from build123d import *

# Parameters (mm, degrees)
SKETCH_1_R                = 30
EXTRUDE_1_DEPTH           = 8
HOLE_WIZARD_2_AT_2_COUNT  = 2
HOLE_WIZARD_2_AT_2_PITCH  = 24
MM_1_D                    = 3
HOLE_WIZARD_3_D           = 4.5
HOLE_WIZARD_3_CBORE_D     = 8
HOLE_WIZARD_3_CBORE_DEPTH = 4.6


with BuildPart() as part:
    # 草图1 → 凸台-拉伸1 (new body)
    with BuildSketch(Plane.XY):
        Circle(SKETCH_1_R)
    extrude(amount=EXTRUDE_1_DEPTH)

    # 草图10 → 打孔尺寸(%根据)内六角圆柱头螺钉的类型2 (revolve, cut)
    with BuildSketch(Plane.YZ.offset(12)):
        Polygon((0, 0), (0, 8), (2.25, 8), (2.25, 4.6), (4, 4.6), (4, 0.025), (4.025, 0), align=None)
    hole_wizard_2 = revolve(axis=Axis((12, 0, -6.35), (0, 0, 1)), mode=Mode.SUBTRACT)

    # 打孔尺寸(%根据)内六角圆柱头螺钉的类型2 at 2: 打孔尺寸(%根据)内六角圆柱头螺钉的类型2 ×2
    with Locations(*[(-i * HOLE_WIZARD_2_AT_2_PITCH, 0, 0) for i in range(1, HOLE_WIZARD_2_AT_2_COUNT)]):
        add(hole_wizard_2, mode=Mode.SUBTRACT)

    # 大小mm 暗销孔1 (through all)
    with Locations(Plane(origin=(0, 0, 0), x_dir=(-1, 0, 0), z_dir=(0, 0, -1))):
        with Locations((0, -17), (0, 17)):
            Hole(MM_1_D / 2)

    # 打孔尺寸(%根据)内六角圆柱头螺钉的类型3 (through all)
    with Locations(Plane.XY.offset(8)):
        with Locations((-20.673237657, 7.524443153), (-20.673237657, -7.524443153), (20.673237657, 7.524443153), (20.673237657, -7.524443153)):
            CounterBoreHole(HOLE_WIZARD_3_D / 2, HOLE_WIZARD_3_CBORE_D / 2, HOLE_WIZARD_3_CBORE_DEPTH)


solid = part.part
Geometry: final body of the model. Coordinates: model frame, mm. A direction names the side the tool comes from. Coordinates: 2 decimals unless noted, no trailing zeros. Write each loop counter-clockwise with the first axis right and the second up, starting at its lowest first coordinate (ties: lowest second). Pieces come first, ordered by that corner, then holes. Notation, with made-up numbers: (-25, 73) - (2, 73) arc R15 cw to (2, 86) - close; hole circle Ø4 at (-25, 7). An arc over 180 degrees is marked (long way). Return JSON: item names as keys, results as strings.
Item 1: Line query: L1, parallel to X at y = 8, z = 3; L2, parallel to X at y = 9.5, z = 1.5; L3, parallel to Y at x = 17, z = 4.75. Output: solid intervals per line, ascending.
Completed:
{"L1": "x = -28.91 to -22.87, -18.47 to 18.47, 22.87 to 28.91", "L2": "x = -28.46 to -21.75, -19.6 to 19.6, 21.75 to 28.46", "L3": "y = -24.72 to -9.11, -5.94 to 5.94, 9.11 to 24.72"}
Item 2: Section query A-A (y = 0). Output: boundary loops of the cut face in (x, z) (3 decimals), and give its area (3 significant figures).
Completed:
{"outline": "(-30, 0) - (-16.025, 0) - (-16, 0.025) - (-16, 4.6) - (-14.25, 4.6) - (-14.25, 8) - (-30, 8) - close; (-9.75, 4.6) - (-8, 4.6) - (-8, 0.025) - (-7.975, 0) - (7.975, 0) - (8, 0.025) - (8, 4.6) - (9.75, 4.6) - (9.75, 8) - (-9.75, 8) - close; (14.25, 4.6) - (16, 4.6) - (16, 0.025) - (16.025, 0) - (30, 0) - (30, 8) - (14.25, 8) - close", "area": "376 mm2"}
Item 3: Reachability of faces 1 (the face through (-15.966, -0.521, 2.28)), 2 (the face through (-16.86, -6.32, 5.73)), 3 (the face through (-0.195, -15.513, 4.056)) from +Z, -Z, +X, -X, +Y, -Y: full face, straight path, thin tool, end or side. Return the list, or none.
Completed:
{"face 1": "-Z", "face 2": "+Z", "face 3": "+Z, -Z"}
Item 4: Section query D-D (x = -12). Output: boundary loops of the cut face in (y, z) (3 decimals).
Completed:
{"outline": "(-27.495, 0) - (-4.025, 0) - (-4, 0.025) - (-4, 4.6) - (-2.25, 4.6) - (-2.25, 8) - (-27.495, 8) - close; (2.25, 4.6) - (4, 4.6) - (4, 0.025) - (4.025, 0) - (27.495, 0) - (27.495, 8) - (2.25, 8) - close"}
Item 5: Section query B-B (x = 0). Output: boundary loops of the cut face in (y, z).
Completed:
{"outline": "(-30, 0) - (-18.5, 0) - (-18.5, 8) - (-30, 8) - close; (-15.5, 0) - (15.5, 0) - (15.5, 8) - (-15.5, 8) - close; (18.5, 0) - (30, 0) - (30, 8) - (18.5, 8) - close"}
Item 6: Pull-direction query (Y, two-part tool) for faces 4 (the face through (22.92, 7.62, 1.68)), 5 (the face through (0, 0, 0)), 6 (the face through (-29.97, 1.32, 3.94)); classes: +Y half, -Y half, draft (parallel to the pull), parting line (faces both ways), or undercut.
Completed:
{"face 4": "undercut", "face 5": "draft", "face 6": "parting line"}
Item 7: Section query C-C (y = 17). Output: boundary loops of the cut face in (x, z).
Completed:
{"outline": "(-24.72, 0) - (-1.5, 0) - (-1.5, 8) - (-24.72, 8) - close; (1.5, 0) - (24.72, 0) - (24.72, 8) - (1.5, 8) - close"}
Item 8: Pin query (flat end, axial travel): pin 1 Ø7 at (x, y) = (20.67, 7.52) entering from +Z; pin 2 Ø1.5 at (y, z) = (6.5, 5) entering from -X. Return the tip coordinate at first contact, or that it passes through.
Completed:
{"pin 1": "stops at z = 3.4", "pin 2": "stops at x = -29.44"}
